from build123d import *
from OCP.BRepFilletAPI import BRepFilletAPI_MakeChamfer

# Parameters (mm, degrees)
SKETCH1_W            = 93.98
SKETCH1_H            = 50.8
BOSS_EXTRUDE1_DEPTH  = 3.175
BOSS_EXTRUDE2_DEPTH  = 3.175
FILLET1_R            = 0.762
BOSS_EXTRUDE3_DEPTH  = 11.43
FILLET2_R            = 1.6002
SKETCH4_W            = 3.175
SKETCH4_H            = 15.24
SKETCH4_H_2          = 3.175
BOSS_EXTRUDE4_DEPTH  = 38.1
CHAMFER1_SIZE        = 15.24
SKETCH8_W            = 19.05
SKETCH8_H            = 17.78
BOSS_EXTRUDE5_DEPTH  = 25.4
SKETCH9_W            = 7.62
SKETCH9_H            = 11.43
CUT_EXTRUDE3_DEPTH   = 110.809108912
CHAMFER2_SIZE        = 3.175
CHAMFER2_SIZE_2      = 25.4
SKETCH14_W           = 17.78
SKETCH14_H           = 22.86
SKETCH14_W_2         = 7.62
SKETCH14_H_2         = 11.43
BOSS_EXTRUDE11_DEPTH = 2.54
SKETCH10_W           = 17.78
SKETCH10_H           = 22.86
SKETCH10_W_2         = 12.7
SKETCH10_H_2         = 17.78
BOSS_EXTRUDE12_DEPTH = 6.35
SKETCH11_W           = 6.35
SKETCH11_H           = 3.175
BOSS_EXTRUDE7_DEPTH  = 14.605
CHAMFER3_SIZE        = 3.175
SKETCH13_W           = 17.78
SKETCH13_H           = 20.6375
BOSS_EXTRUDE8_DEPTH  = 2.54
CHAMFER4_SIZE        = 3.175
SKETCH15_W           = 93.98
SKETCH15_H           = 15.24
BOSS_EXTRUDE13_DEPTH = 3.175
CHAMFER5_SIZE        = 3.175
CHAMFER5_SIZE_2      = 50.8
SKETCH17_W           = 26.67
SKETCH17_H           = 14.605
BOSS_EXTRUDE14_DEPTH = 3.175


# Some blends are built 0.0001 mm under size
with BuildPart() as part:
    # Sketch1 → Boss-Extrude1 (new body)
    with BuildSketch(Plane(origin=(0, 0, 0), x_dir=(1, 0, 0), z_dir=(0, 1, 0))):
        with Locations((46.99, 25.4)):
            Rectangle(SKETCH1_W, SKETCH1_H)
    extrude(amount=BOSS_EXTRUDE1_DEPTH)

    # Sketch2 → Boss-Extrude2 (add)
    with BuildSketch(Plane.XY.offset(-19.05)):
        with BuildLine():
            Line((87.63, 3.175), (13.127130217, 13.221093478))
            ThreePointArc((13.127130217, 13.221093478), (12.280474231, 13.306491372), (11.43, 13.335))
            Line((11.43, 13.335), (-26.67, 13.335))
            Line((-26.67, 13.335), (-26.67, 3.175))
            Line((-26.67, 3.175), (87.63, 3.175))
        make_face()
    extrude(amount=BOSS_EXTRUDE2_DEPTH)

    # Fillet1
    fillet1_edges = [part.edges().sort_by_distance(p)[0] for p in [
        (50.378565109, 8.198046739, -19.05),
        (12.280474231, 13.306491372, -19.05),
        (-7.62, 13.335, -19.05),
        (50.378565109, 8.198046739, -15.875),
        (12.280474231, 13.306491372, -15.875),
        (-7.62, 13.335, -15.875),
    ]]
    fillet(fillet1_edges, radius=FILLET1_R)

    # Sketch3 → Boss-Extrude3 (add)
    with BuildSketch(Plane(origin=(0, 3.175, 0), x_dir=(1, 0, 0), z_dir=(0, 1, 0))):
        Polygon((43.18, 10.45493597), (40.93493597, 12.7), (18.484295667, -9.750640303), (20.729359697, -11.995704333), align=None)
    extrude(amount=BOSS_EXTRUDE3_DEPTH)

    # Fillet2
    # the kernel refuses this fillet: 1.6002 mm, written as the material it takes off along each edge
    with BuildSketch(Plane(origin=(40.93493597, 3.175, -12.7), x_dir=(0.7071067811865515, 0, 0.7071067811865437), z_dir=(0, 1, 0)), Plane(origin=(43.18, 3.175, -10.45493597), x_dir=(-0.7071067811865437, 0, 0.7071067811865515), z_dir=(0, 1, 0))) as fillet2_piece_1:
        with BuildLine():
            CenterArc((FILLET2_R, -FILLET2_R), FILLET2_R, 90, 90)
            Line((0, -FILLET2_R), (0, 0))
            Line((0, 0), (FILLET2_R, 0))
        make_face()
    extrude(amount=15.4305, mode=Mode.SUBTRACT)

    # Sketch4 → Boss-Extrude4 (add)
    with BuildSketch(Plane.ZY):
        with Locations((-24.765, 10.795)):
            Rectangle(SKETCH4_W, SKETCH4_H)
        with Locations((-10.16, 10.795)):
            Rectangle(SKETCH4_W, SKETCH4_H)
        with Locations((-10.16, 1.5875)):
            Rectangle(SKETCH4_W, SKETCH4_H_2)
        with Locations((-24.765, 1.5875)):
            Rectangle(SKETCH4_W, SKETCH4_H_2)
    extrude(amount=BOSS_EXTRUDE4_DEPTH)

    # Chamfer1
    chamfer1_edges = [part.edges().sort_by_distance(p)[0] for p in [
        (0, 3.175, -10.16),
        (0, 3.175, -24.765),
    ]]
    chamfer(chamfer1_edges, length=CHAMFER1_SIZE - 0.0001)  # a hair under: the kernel refuses the full size

    # Sketch8 → Boss-Extrude5 (add)
    with BuildSketch(Plane.XZ):
        with Locations((-28.575, -17.4625)):
            Rectangle(SKETCH8_W, SKETCH8_H)
    extrude(amount=BOSS_EXTRUDE5_DEPTH)

    # Sketch9 → Cut-Extrude3 (cut, through all)
    with BuildSketch(Plane(origin=(0, 0, 0), x_dir=(1, 0, 0), z_dir=(0, 1, 0))):
        with Locations((-31.115, 17.4625)):
            Rectangle(SKETCH9_W, SKETCH9_H)
    extrude(amount=-CUT_EXTRUDE3_DEPTH, mode=Mode.SUBTRACT)

    # Chamfer2
    chamfer2_edges_1 = [part.edges().sort_by_distance(p)[0] for p in [
        (-27.305, 0, -17.4625),
    ]]
    chamfer2_side_1 = [part.faces().sort_by_distance(p)[0] for p in [
        (-27.2415, 0, -17.4625),
    ]]
    chamfer2_edges_2 = [part.edges().sort_by_distance(p)[0] for p in [
        (-34.925, 0, -17.4625),
    ]]
    chamfer2_side_2 = [part.faces().sort_by_distance(p)[0] for p in [
        (-34.9885, 0, -17.4625),
    ]]
    chamfer2 = BRepFilletAPI_MakeChamfer(part.part.solid().wrapped)
    for e in chamfer2_edges_1:
        chamfer2.Add(CHAMFER2_SIZE - 0.0001, CHAMFER2_SIZE_2 - 0.0001, e.wrapped, chamfer2_side_1[0].wrapped)
    for e in chamfer2_edges_2:
        chamfer2.Add(CHAMFER2_SIZE - 0.0001, CHAMFER2_SIZE_2 - 0.0001, e.wrapped, chamfer2_side_2[0].wrapped)
    add(Compound.cast(chamfer2.Shape()), mode=Mode.REPLACE)  # a hair under: the kernel refuses the full size

    # Sketch14 → Boss-Extrude11 (add)
    with BuildSketch(Plane.XZ.offset(25.4)):
        with Locations((-31.115, -17.4625)):
            Rectangle(SKETCH14_W, SKETCH14_H)
        with Locations((-31.115, -17.4625)):
            Rectangle(SKETCH14_W_2, SKETCH14_H_2, mode=Mode.SUBTRACT)
    extrude(amount=-BOSS_EXTRUDE11_DEPTH)

    # Sketch10 → Boss-Extrude12 (add)
    with BuildSketch(Plane.XZ.offset(25.4)):
        with Locations((-31.115, -17.4625)):
            Rectangle(SKETCH10_W, SKETCH10_H)
        with Locations((-31.115, -17.4625)):
            Rectangle(SKETCH10_W_2, SKETCH10_H_2, mode=Mode.SUBTRACT)
    extrude(amount=BOSS_EXTRUDE12_DEPTH)

    # Sketch11 → Boss-Extrude7 (add)
    with BuildSketch(Plane(origin=(0, 0, -11.7475), x_dir=(-1, 0, 0), z_dir=(0, 0, -1))):
        with Locations((34.925, 16.8275)):
            Rectangle(SKETCH11_W, SKETCH11_H)
    extrude(amount=BOSS_EXTRUDE7_DEPTH)

    # Chamfer3
    chamfer3_edges = [part.edges().sort_by_distance(p)[0] for p in [
        (-31.75, 15.24, -17.4625),
    ]]
    chamfer(chamfer3_edges, length=CHAMFER3_SIZE - 0.0001)  # a hair under: the kernel refuses the full size

    # Sketch13 → Boss-Extrude8 (add)
    with BuildSketch(Plane.ZY.offset(38.1)):
        with Locations((-17.4625, 8.09625)):
            Rectangle(SKETCH13_W, SKETCH13_H)
    extrude(amount=BOSS_EXTRUDE8_DEPTH)

    # Chamfer4
    # the kernel refuses this chamfer: 3.175 mm, written as the material it adds along each edge
    with BuildSketch(Plane(origin=(-38.1, -2.2225, -8.5725), x_dir=(0.02749587661058565, -0.9996219169112968, 0), z_dir=(0, 0, -1))) as chamfer4_piece_1_section:
        Polygon((CHAMFER4_SIZE * 0.999621916911, CHAMFER4_SIZE * 0.0274958766106), (-CHAMFER4_SIZE * 0.0274958766106, CHAMFER4_SIZE * 0.999621916911), (0, 0), align=None)
    chamfer4_piece_1 = extrude(amount=17.78, mode=Mode.PRIVATE)
    chamfer4_piece_1 = split(chamfer4_piece_1, bisect_by=Plane(origin=(-40.64, -3.320155959, -17.4625), z_dir=(1, 0, 0)), keep=Keep.TOP, mode=Mode.PRIVATE)
    add(chamfer4_piece_1)

    # Sketch15 → Boss-Extrude13 (add)
    with BuildSketch(Plane(origin=(0, 0, -26.3525), x_dir=(-1, 0, 0), z_dir=(0, 0, -1))):
        with Locations((-46.99, 10.795)):
            Rectangle(SKETCH15_W, SKETCH15_H)
    extrude(amount=-BOSS_EXTRUDE13_DEPTH)

    # Chamfer5
    # the kernel refuses this chamfer: 50.8, 3.175 mm, written as the material it takes off along each edge
    with BuildSketch(Plane(origin=(93.98, 150.485487252, -23.1775), x_dir=(0.5233850041899423, 0, -0.8520963193143684), z_dir=(0, -1, 0))) as chamfer5_piece_1:
        Polygon((CHAMFER5_SIZE * 0.852096319314, -CHAMFER5_SIZE * 0.52338500419), (-CHAMFER5_SIZE_2 * 0.52338500419, -CHAMFER5_SIZE_2 * 0.852096319314), (0, 0), align=None)
    extrude(amount=147.310487252, mode=Mode.SUBTRACT)

    # Sketch17 → Boss-Extrude14 (add)
    with BuildSketch(Plane.XZ.offset(-3.175)):
        with Locations((-13.335, -19.05)):
            Rectangle(SKETCH17_W, SKETCH17_H)
    extrude(amount=BOSS_EXTRUDE14_DEPTH)


solid = part.part
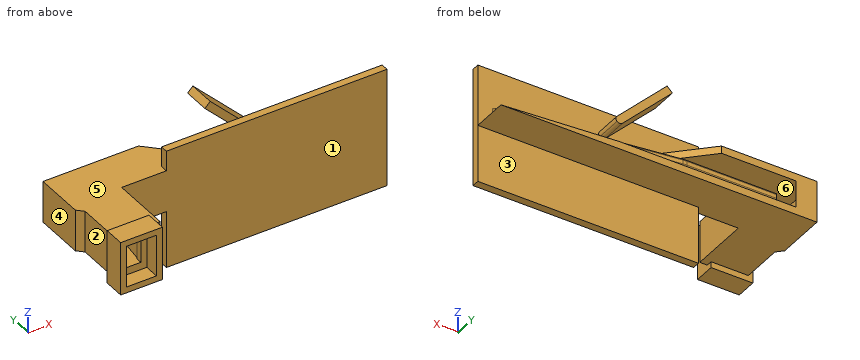
Verification items for the finished model (mm, model axes). Face numbers are marked on the shaded views. A direction names the side the tool comes from. Give positions to 0.01 mm unless a question says otherwise; leave off trailing zeros. Loops run counter-clockwise (first coordinate to the right, second up) from the corner with the lowest first, then second, coordinate; pieces in that order, holes last.
1. Release check for a two-part mould opening along X. For the marked faces 4, 5 and 6 record: +X half, -X half, draft (parallel to the pull), parting line (faces both ways), or undercut.
Derived:
face 4: -X half
face 5: draft
face 6: undercut
2. Go/stop test with flat-tipped pins: P1, Ø7, axis at x = -30.5, y = -28, coming from the +Z side; P2, Ø9.5, axis at x = 23, z = 8.5, coming from the -Y side (3 decimals); P3, Ø4.5, axis at x = 39, y = 8, coming from the -Z side. Record where each tip stops, or that it passes through.
Derived:
P1: stops at z = -6.03
P2: stops at y = 3.175
P3: stops at z = -26.35
3. Cross-section at C-C on z = -32. Record the cut outline in (x, y) (3 decimals), and give its area (3 significant figures).
Derived:
outline: (0, 0) - (93.98, 0) - (93.98, 3.175) - (0, 3.175) - close
area: 298 mm2
4. Tool access check on the marked faces 1, 2 and 3. Record the directions out of +Z, -Z, +X, -X, +Y, -Y that give a thin tool (end or side, any length) a straight path to the whole face; none if there is none.
Derived:
face 1: +Z, -Z, +X, -Y
face 2: +Z, -Z, -X
face 3: -Z, +X, -X, +Y
5. Material ranges on probe 1 along X at (y, z) = (-27, -15) (3 decimals); probe 2 along Y at (x, z) = (-32, -26.5); probe 3 along Z at (x, y) = (-3.5, 15.5), recorded low to high.
Derived:
probe 1: x = -40.005 to -37.465, -24.765 to -22.225
probe 2: y = -31.75 to -22.86
probe 3: z = -26.35 to -23.18, -11.75 to -8.57
6. Cross-section at D-D on y = -18. Record the cut outline in (x, z), and give its area (3 significant figures).
Derived:
outline: (-38.1, -26.35) - (-19.05, -26.35) - (-19.05, -8.57) - (-38.1, -8.57) - close; hole (-35.85, -23.18) - (-26.38, -23.18) - (-26.38, -11.75) - (-35.85, -11.75) - close
area: 230 mm2
7. Cross-section at A-A on y = 1.5. Record the cut outline in (x, z).
Derived:
outline: (-40.64, -26.35) - (0, -26.35) - (0, -50.8) - (93.98, -50.8) - (93.98, 0) - (0, 0) - (0, -8.57) - (-40.64, -8.57) - close; hole (-38.1, -23.18) - (-26.67, -23.18) - (-26.67, -11.75) - (-38.1, -11.75) - close
